Here's how the part is built. I have some questions about the finished solid (model axes, mm). A direction names the side the tool comes from. Round coordinates to 2 decimals unless told otherwise and drop trailing zeros. Write each loop counter-clockwise with the first axis right and the second up, starting at its lowest first coordinate (ties: lowest second). Pieces come first, ordered by that corner, then holes. Notation, with made-up numbers: (-11.5, 41) -> (36.5, 41) arc R19 ccw to (36.5, 63) -> close; hole circle Ø1 at (85.5, 11.25). An arc over 180 degrees is marked (long way). Put each result on its own line as item: value. Start each with the question number.
1. We'd pull the mould along X, two halves only. Please class faces 6 (the face through (0, -12, -3)), 7 (the face through (0.325, -16.964, -1.507)), 8 (the face through (-11.311, 6.958, 6.404)), 9 (the face through (-2.4, -11.4, 3.2)): +X half, -X half, draft (parallel to the pull), parting line (faces both ways), or undercut.
2. Suppose I cut it at D-D (x = 4.5). Please give me the cut outline in (y, z), then the cut area to 3 significant figures.
3. Suppose I cut it at A-A (x = 0). Please give me the cut outline in (y, z), then the cut area to 3 significant figures.
4. Suppose I cut it at B-B (z = 0). Please give me the cut outline in (x, y).
5. I need wall thicknesses on probe 1 along Y at (x, z) = (0, -1.45); probe 2 along Y at (x, z) = (3.75, 0.5); probe 3 along X at (y, z) = (-2.5, 0.25). Which ranges of each line are inside material? Lowest first, please. Write a range as from..to.
6. For pin 1 (0.6 mm diameter, centred on x = 0, z = -3, fed in from -Y); pin 2 (8 mm diameter, centred on y = 1.5, z = -5.5, fed in from -X); pin 3 (0.9 mm diameter, centred on x = -0.5, y = -15.5, fed in from -Z), each with a flat end and sliding along its axis, tell me the tip position at first contact or that it passes through.
7. Suppose I cut it at C-C (y = -15.5). Please give me the cut outline in (x, z), then the cut area to 3 significant figures.
8. Which directions (+Z, -Z, +X, -X, +Y, -Y) give clear straight access to the entire face, cutting with the end or side of a thin tool? Please do faces 1 (the face through (-1, -17, -2)), 2 (the face through (9, 10, 5)), 3 (the face through (6.875, 6.958, 6.404)), 4 (the face through (0, -15, -1)), 5 (the face through (5.37, -0.49, -1.19)).
```python
from build123d import *

# Parameters (mm, degrees)
SKETCH_1_R          = 13.5
EXTRUDE_1_DEPTH     = 4
SKETCH_2_R          = 2.5
EXTRUDE_2_DEPTH     = 6
SKETCH_3_R          = 4
EXTRUDE_3_DEPTH     = 7
SKETCH_4_R          = 5.5
EXTRUDE_4_DEPTH     = 1
SKETCH_5_R          = 4
EXTRUDE_5_DEPTH     = 15
CUT_EXTRUDE_START   = -10
CUT_EXTRUDE_1_DEPTH = 10
SKETCH_7_R          = 1.5
CUT_EXTRUDE_2_DEPTH = 1


with BuildPart() as part:
    # 草图1 → 凸台-拉伸1 (new body)
    with BuildSketch(Plane(origin=(0, 0, 0), x_dir=(1, 0, 0), z_dir=(0, 1, 0))):
        with Locations(Location((0, 0, 0), (0, 0, 270))):
            Circle(SKETCH_1_R)
    extrude(amount=EXTRUDE_1_DEPTH)

    # 草图2 → 凸台-拉伸2 (add)
    with BuildSketch(Plane(origin=(0, 4, 0), x_dir=(1, 0, 0), z_dir=(0, 1, 0))):
        with Locations(Location((0, 10.5, 0), (0, 0, 270))):
            Circle(SKETCH_2_R)
        with Locations(Location((9.09326674, -5.25, 0), (0, 0, 270))):
            Circle(SKETCH_2_R)
        with Locations(Location((-9.09326674, -5.25, 0), (0, 0, 270))):
            Circle(SKETCH_2_R)
    extrude(amount=EXTRUDE_2_DEPTH)

    # 草图3 → 凸台-拉伸3 (add)
    with BuildSketch(Plane.XZ):
        with Locations(Location((0, 0, 0), (0, 0, 270))):
            Circle(SKETCH_3_R)
    extrude(amount=EXTRUDE_3_DEPTH)

    # 草图4 → 凸台-拉伸4 (add)
    with BuildSketch(Plane.XZ):
        with Locations(Location((0, 0, 0), (0, 0, 90))):
            Circle(SKETCH_4_R)
    extrude(amount=EXTRUDE_4_DEPTH)

    # 草图5 → 凸台-拉伸5 (add)
    with BuildSketch(Plane.XZ.offset(7)):
        with Locations(Location((0, 0, 0), (0, 0, 270))):
            Circle(SKETCH_5_R)
    extrude(amount=EXTRUDE_5_DEPTH)

    # 草图6 → 切除-拉伸1 (cut)
    with BuildSketch(Plane.XZ.offset(22).offset(CUT_EXTRUDE_START)):
        with BuildLine():
            Line((3.464101615, -2), (-3.464101615, -2))
            ThreePointArc((-3.464101615, -2), (0, -4), (3.464101615, -2))
        make_face()
    extrude(amount=CUT_EXTRUDE_1_DEPTH, mode=Mode.SUBTRACT)

    # 草图7 → 切除-拉伸2 (cut)
    with BuildSketch(Plane(origin=(0, 0, -2), x_dir=(-1, 0, 0), z_dir=(0, 0, -1))):
        with Locations((0, -15.5)):
            Circle(SKETCH_7_R)
    extrude(amount=-CUT_EXTRUDE_2_DEPTH, mode=Mode.SUBTRACT)


solid = part.part
```
Verdict:
1. face 6: draft
1. face 7: undercut
1. face 8: undercut
1. face 9: parting line
2. outline: (-1, -3.16) -> (0, -3.16) -> (0, -12.73) -> (4, -12.73) -> (4, 12.73) -> (0, 12.73) -> (0, 3.16) -> (-1, 3.16) -> close
2. area: 108 mm^2
3. outline: (-22, -2) -> (-17, -2) -> (-17, -1) -> (-14, -1) -> (-14, -2) -> (-12, -2) -> (-12, -4) -> (-1, -4) -> (-1, -5.5) -> (0, -5.5) -> (0, -13.5) -> (4, -13.5) -> (4, -13) -> (10, -13) -> (10, -8) -> (4, -8) -> (4, 13.5) -> (0, 13.5) -> (0, 5.5) -> (-1, 5.5) -> (-1, 4) -> (-22, 4) -> close
3. area: 294 mm^2
4. outline: (-13.5, 0) -> (-5.5, 0) -> (-5.5, -1) -> (-4, -1) -> (-4, -22) -> (4, -22) -> (4, -1) -> (5.5, -1) -> (5.5, 0) -> (13.5, 0) -> (13.5, 4) -> (-13.5, 4) -> close
5. probe 1: y = -22..-17, -14..4
5. probe 2: y = -22..4
5. probe 3: x = -3.99..3.99
6. pin 1: stops at y = -12
6. pin 2: stops at x = -13.42
6. pin 3: stops at z = -1
7. outline: (-3.46, -2) -> (-1.5, -2) -> (-1.5, -1) -> (1.5, -1) -> (1.5, -2) -> (3.46, -2) arc R4 ccw (long way) to start
7. area: 37.4 mm^2
8. face 1: -Z, +X, -X, -Y
8. face 2: +Z, -Z, +X, -X, +Y
8. face 3: +Y
8. face 4: -Z
8. face 5: -Y
